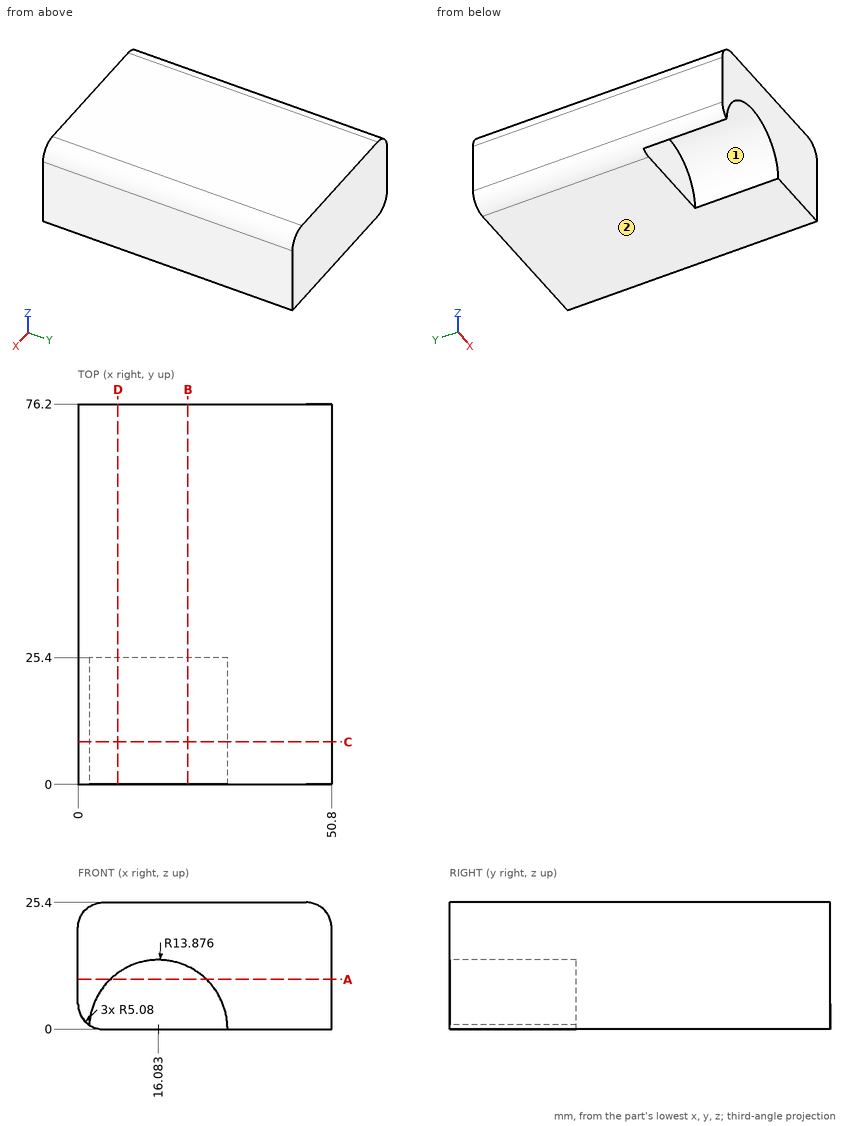
The figure shows three views and two pictorial views of one solid part (mm, origin at its lowest corner). Answer the questions. A direction names the side the tool comes from. Coordinates: 2 decimals unless noted, no trailing zeros. Loops run counter-clockwise (first coordinate to the right, second up) from the corner with the lowest first, then second, coordinate; pieces in that order, holes last. Notation, with made-up numbers: (12, -7) -> (40, -7) arc R29 cw to (40, 28) -> close; hole circle Ø7 at (75.25, 63). An arc over 180 degrees is marked (long way). Use one line per item in the form item = value. Start each with the question number.
Item 1: A tool of negligible diameter and unlimited length cuts with its end or side. For the marked faces 1 and 2, from which of +Z, -Z, +X, -X, +Y, -Y can it reach the whole face along a straight path? Write none if from no direction.
Item 2: The part is cut by section A-A on z = 10. Determine the outline of the cut face in (x, y).
Item 3: The part is cut by section B-B on x = 22. Determine the outline of the cut face in (y, z).
Item 4: The part is cut by section C-C on y = 8.5. Determine the outline of the cut face in (x, z) (1 decimal), then the cut area to 3 significant figures.
Item 5: The part is cut by section D-D on x = 8. Determine the outline of the cut face in (y, z).
Item 6: Consider L1, parallel to Y at x = 4, z = 2.5; L2, parallel to Z at x = 15.5, y = 25; L3, parallel to Z at x = 22.5, y = 18. Determine where each line is inside the solid, lowest interval first. Write a range as [from, to].
Answer key:
q1.face_1 = -Z, -Y
q1.face_2 = -Z, +X, -X, +Y, -Y
q2.outline = (0, 0) -> (6.46, 0) -> (6.46, 25.4) -> (25.7, 25.4) -> (25.7, 0) -> (50.8, 0) -> (50.8, 76.2) -> (0, 76.2) -> close
q3.outline = (0, 12.55) -> (25.4, 12.55) -> (25.4, 0) -> (76.2, 0) -> (76.2, 25.4) -> (0, 25.4) -> close
q4.outline = (0, 5.1) arc R5.1 ccw to (2.2, 0.9) arc R13.9 cw to (30, 0) -> (50.8, 0) -> (50.8, 20.3) arc R5.1 ccw to (45.7, 25.4) -> (5.1, 25.4) arc R5.1 ccw to (0, 20.3) -> close
q4.area = 972 mm2
q5.outline = (0, 11.28) -> (25.4, 11.28) -> (25.4, 0) -> (76.2, 0) -> (76.2, 25.4) -> (0, 25.4) -> close
q6.L1 = [25.4, 76.2]
q6.L2 = [13.86, 25.4]
q6.L3 = [12.3, 25.4]
